from build123d import *
from OCP.BRepFilletAPI import BRepFilletAPI_MakeChamfer

# Parameters (mm, degrees)
CHAMFER1_SIZE      = 0.4
CHAMFER1_SIZE2     = 0.230940108
SKETCH2_R          = 2.5
CUT_EXTRUDE1_DEPTH = 16.305227865
SKETCH3_R          = 4
SKETCH3_R_2        = 3.25
CUT_EXTRUDE2_DEPTH = 0.5
CUT_EXTRUDE3_START = -0.5
SKETCH4_R          = 4
SKETCH4_R_2        = 3.25
CUT_EXTRUDE3_DEPTH = 0.5


with BuildPart() as part:
    # Sketch1 → Revolve1 (revolve)
    with BuildSketch(Plane.XY, mode=Mode.PRIVATE) as revolve1_sk:
        Polygon((0, 0), (0, 9), (1, 9), (1, 6), (7.5, 6), (7.5, 9), (8.5, 9), (8.5, 0), align=None)
    revolve(revolve1_sk.sketch.rotate(Axis((0, 0, 0), (1, 0, 0)), 90), axis=Axis((0, 0, 0), (1, 0, 0)))

    # Chamfer1: one chamfer whose edges measure the first distance from different faces: ONE call of the kernel's chamfer builder (chamfer() names one face for all edges)
    chamfer1_edges_1 = [part.edges().sort_by_distance(p)[0] for p in [
        (8.5, 0, -9),
    ]]
    chamfer1_side_1 = [part.faces().sort_by_distance(p)[0] for p in [
        (8.5, 0, 0),
    ]]
    chamfer1_edges_2 = [part.edges().sort_by_distance(p)[0] for p in [
        (0, 0, -9),
    ]]
    chamfer1_side_2 = [part.faces().sort_by_distance(p)[0] for p in [
        (0.5, 0, -9),
    ]]
    chamfer1 = BRepFilletAPI_MakeChamfer(part.part.solid().wrapped)
    for e in chamfer1_edges_1:
        chamfer1.Add(CHAMFER1_SIZE, CHAMFER1_SIZE2, e.wrapped, chamfer1_side_1[0].wrapped)  # the first distance lies on this face
    for e in chamfer1_edges_2:
        chamfer1.Add(CHAMFER1_SIZE, CHAMFER1_SIZE2, e.wrapped, chamfer1_side_2[0].wrapped)  # the first distance lies on this face
    add(Compound.cast(chamfer1.Shape()), mode=Mode.REPLACE)

    # Sketch2 → Cut-Extrude1 (cut, through all)
    with BuildSketch(Plane(origin=(8.5, 0, 0), x_dir=(0, 0, -1), z_dir=(1, 0, 0))):
        Circle(SKETCH2_R)
    extrude(amount=-CUT_EXTRUDE1_DEPTH, mode=Mode.SUBTRACT)

    # Sketch3 → Cut-Extrude2 (cut)
    with BuildSketch(Plane(origin=(8.5, 0, 0), x_dir=(0, 0, -1), z_dir=(1, 0, 0))):
        Circle(SKETCH3_R)
        Circle(SKETCH3_R_2, mode=Mode.SUBTRACT)
    extrude(amount=-CUT_EXTRUDE2_DEPTH, mode=Mode.SUBTRACT)

    # Sketch4 → Cut-Extrude3 (cut)
    with BuildSketch(Plane.ZY.offset(CUT_EXTRUDE3_START)):
        with Locations(Location((0, 0, 0), (0, 0, 180))):
            Circle(SKETCH4_R)
        with Locations(Location((0, 0, 0), (0, 0, 180))):
            Circle(SKETCH4_R_2, mode=Mode.SUBTRACT)
    extrude(amount=CUT_EXTRUDE3_DEPTH, mode=Mode.SUBTRACT)


solid = part.part
Geometry check sheet. Reference: the model listing, model coordinates, mm. A direction names the side the tool comes from. Give positions to 0.01 mm unless a question says otherwise; leave off trailing zeros. Order: outer loops, then holes, each group sorted by start corner. A loop starts at its lowest first (then second) coordinate and runs counter-clockwise, first axis right, second up. Notation, with made-up numbers: (-16, 64.5) - (41, 64.5) arc R24 ccw to (41, 97.5) - close; hole circle Ø3 at (66, 53.25). An arc over 180 degrees is marked (long way). Use one line per item in the form item = value.
1) Access from +Z, -Z, +X, -X, +Y, -Y to the whole of each face (thin tool, end or side, straight path). Record for faces 4 (the face through (0.704, -6.083, -6.633)), 5 (the face through (1, 6, 2)), 6 (the face through (8, 3, 2)), 7 (the face through (0, 2, -2)), 8 (the face through (0.5, -3, 2)).
Working result:
face_4 = +X, -X
face_5 = none
face_6 = +X
face_7 = +Z, -Z, -X, +Y, -Y
face_8 = -X
2) Depth check by flat-ended pin: pin 1 Ø3 at (x, z) = (4, 6.5) entering from -Y; pin 2 Ø2 at (x, y) = (4.5, 4) entering from +Z. Enter the tip coordinate at first touch or a pass-through.
Working result:
pin_1 = -3.32
pin_2 = 5.2
3) Draft check along X on faces 1 (the face through (8.5, 4, 2)), 2 (the face through (4.296, -1.802, 5.723)), 3 (the face through (0, 4, -2)). Enter one of: released by +X, released by -X, zero draft, split by the parting line, or undercut.
Working result:
face_1 = released by +X
face_2 = undercut
face_3 = released by -X
4) Sectioned sample at A-A (x = 4). Record the boundary of the cut face in (y, z).
Working result:
outline = circle Ø12 at (0, 0); hole circle Ø5 at (0, 0)
5) Material ranges on probe 1 along Y at (x, z) = (0.45, 0); probe 2 along Y at (x, z) = (6.25, 0); probe 3 along X at (y, z) = (-0.5, -7.5), recorded low to high. Write a range as from..to.
Working result:
probe_1 = -9..-4, -3.25..-2.5, 2.5..3.25, 4..9
probe_2 = -6..-2.5, 2.5..6
probe_3 = 0..1, 7.5..8.5
